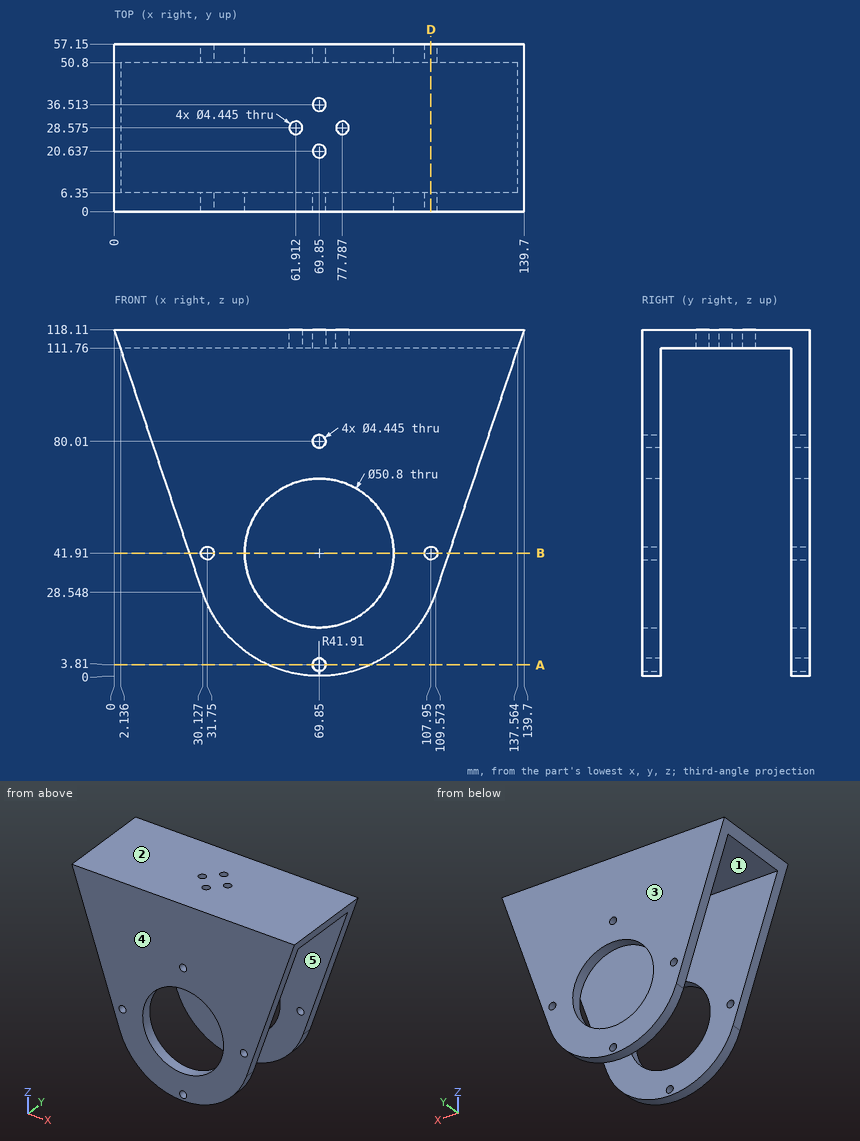
Can you work these out from the drawing? Everything is in mm from the part's minimum corner. A direction names the side the tool comes from. Coordinates: 2 decimals unless noted, no trailing zeros. Write each loop counter-clockwise with the first axis right and the second up, starting at its lowest first coordinate (ties: lowest second). Pieces come first, ordered by that corner, then holes. Notation, with made-up numbers: (71, 14.25) -> (92, 14.25) arc R13 ccw to (92, 18.25) -> close; hole circle Ø10 at (15, -19). An arc over 180 degrees is marked (long way). Return JSON: item names as keys, results as strings.
(1) Imagine slicing it at D-D, the plane x = 107.95. Please give me the cut outline in (y, z).
Numbers:
{"outline": "(0, 24.45) -> (6.35, 24.45) -> (6.35, 39.69) -> (0, 39.69) -> close; (0, 44.13) -> (6.35, 44.13) -> (6.35, 111.76) -> (50.8, 111.76) -> (50.8, 44.13) -> (57.15, 44.13) -> (57.15, 118.11) -> (0, 118.11) -> close; (50.8, 24.45) -> (57.15, 24.45) -> (57.15, 39.69) -> (50.8, 39.69) -> close"}
(2) We'd pull the mould along Y, two halves only. Please class the marked faces 3, 4 and 5: +Y half, -Y half, draft (parallel to the pull), parting line (faces both ways), or undercut.
Numbers:
{"face 3": "+Y half", "face 4": "-Y half", "face 5": "undercut"}
(3) Which directions (+Z, -Z, +X, -X, +Y, -Y) give clear straight access to the entire face, cutting with the end or side of a thin tool? Please do the marked faces 1 and 2.
Numbers:
{"face 1": "-Z, +X, -X", "face 2": "+Z, +X, -X, +Y, -Y"}
(4) Imagine slicing it at A-A, the plane z = 3.81. Please give me the cut outline in (x, y), then the cut area to 3 significant figures.
Numbers:
{"outline": "(52.39, 0) -> (67.63, 0) -> (67.63, 6.35) -> (52.39, 6.35) -> close; (52.39, 50.8) -> (67.63, 50.8) -> (67.63, 57.15) -> (52.39, 57.15) -> close; (72.07, 0) -> (87.31, 0) -> (87.31, 6.35) -> (72.07, 6.35) -> close; (72.07, 50.8) -> (87.31, 50.8) -> (87.31, 57.15) -> (72.07, 57.15) -> close", "area": "387 mm2"}
(5) I'm going to push flat-ended pins straight in: pin 1 (7 mm diameter, centred on x = 69.85, y = 36.51, fed in from -Z); pin 2 (4 mm diameter, centred on x = 31.75, z = 41.91, fed in from -Y); pin 3 (12 mm diameter, centred on y = 6, z = 80.5, fed in from +X); pin 4 (3 mm diameter, centred on y = 6, z = 31, fed in from +X). Where does each tip first touch, or does it pass through?
Numbers:
{"pin 1": "stops at z = 111.76", "pin 2": "passes through", "pin 3": "stops at x = 129.07", "pin 4": "stops at x = 110.9"}
(6) Imagine slicing it at B-B, the plane z = 41.91. Count the separate pieces of the cut face and the enclosed holes in it, then the cut area to 3 significant figures.
Numbers:
{"separate pieces": "8", "enclosed holes": "0", "area": "365 mm2"}
(7) I need wall thicknesses on L1, parallel to Y at x = 52, z = 103; L2, parallel to X at y = 54, z = 41 (1 decimal). Which ranges of each line are inside material? Lowest first, please.
Numbers:
{"L1": "y = 0 to 6.35, 50.8 to 57.15", "L2": "x = 25.9 to 29.7, 33.8 to 44.5, 95.2 to 105.9, 110 to 113.8"}
